For this review, take the finished solid that the model builds, in its own axes (mm). Face numbers are marked on the shaded views. A direction names the side the tool comes from. Coordinates: 2 decimals unless noted, no trailing zeros. Write each loop counter-clockwise with the first axis right and the second up, starting at its lowest first coordinate (ties: lowest second). Pieces come first, ordered by that corner, then holes. Notation, with made-up numbers: (6, 23.25) -> (33, 23.25) arc R20 ccw to (33, 57.25) -> close; hole circle Ø11 at (79, 35). An arc over 180 degrees is marked (long way). Put each result on its own line as item: value. Start each with the question number.
Item 1: Consider section B-B on x = 0. Give the boundary of the cut face in (y, z) (3 decimals), and give its area (3 significant figures).
Item 2: Consider section C-C on x = 23.5. Give the number of separate pieces and of enclosed holes in the cut face, and give its area (3 significant figures).
Item 3: Consider section A-A on y = 37.5. Give the boundary of the cut face in (x, z).
Item 4: Insertion check: P1, Ø8.5, axis at y = 24, z = 24, coming from the -X side; P2, Ø2.5, axis at x = -23.622, z = 23.622, coming from the +Y side; P3, Ø1, axis at x = -13.5, y = 37, coming from the +Z side; P4, Ø2.5, axis at x = -23, z = -24.5, coming from the +Y side. Each pin has a flat end and moves straight along its axis. Give the tip position at first contact, or say it passes through.
Item 5: To check wall thickness, follow L1, parallel to Z at x = 0, y = -0.9 (3 decimals); L2, parallel to Y at x = -16.5, z = 12.5; L3, parallel to X at y = 28.5, z = 24. State the ranges of each line that lie inside material, in increasing order.
Item 6: For the marked faces 1, 2 and 3, list the 3-axis set-ups (+Z, -Z, +X, -X, +Y, -Y) from which the entire face can be reached by the end or side of a thin tool; tool diameter is ignored.
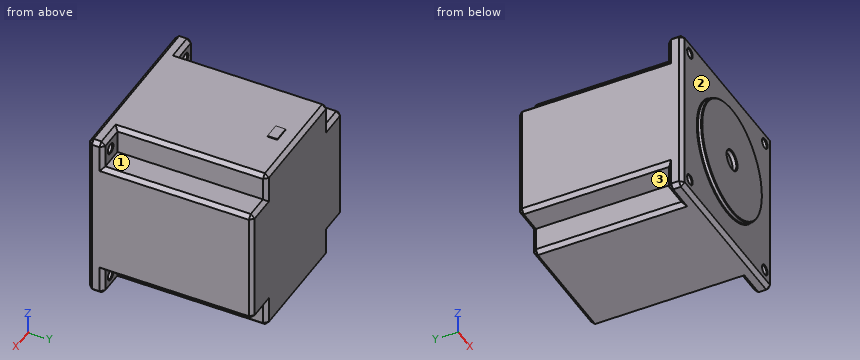
```python
from build123d import *

# Parameters (mm, degrees)
F0_W      = 56.388
F0_H      = 56.388
F0_R      = 1.4859
F0_R_2    = 19.05
F0_R_3    = 3.175
F1_DEPTH  = 54.102
F2_DEPTH  = 1.524
F3_DEPTH  = 20.32
F5_DEPTH  = 12.7
F6_W      = 8.89
F6_H      = 8.89
F7_DEPTH  = 49.022
F8_SIZE   = 1.27
F9_SIZE   = 0.254
F9_2_SIZE = 0.254
F10_W     = 5.2164322697
F10_H     = 3.265157342
F11_DEPTH = 0.254


with BuildPart() as f1:
    # F0 (on Front) → F1 (new body)
    with BuildSketch(Plane.XZ):
        Rectangle(F0_W, F0_H)
        with Locations((-23.622, -23.622)):
            Circle(F0_R, mode=Mode.SUBTRACT)
        with Locations((23.622, -23.622)):
            Circle(F0_R, mode=Mode.SUBTRACT)
        with Locations((-23.622, 23.622)):
            Circle(F0_R, mode=Mode.SUBTRACT)
        Circle(F0_R_2, mode=Mode.SUBTRACT)
        with Locations((23.622, 23.622)):
            Circle(F0_R, mode=Mode.SUBTRACT)
        Circle(F0_R_2)
        Circle(F0_R_3, mode=Mode.SUBTRACT)
        Circle(F0_R_3)
    extrude(amount=-F1_DEPTH)

    # F0 (on Front) → F2 (join)
    with BuildSketch(Plane.XZ):
        Circle(F0_R_2)
        Circle(F0_R_3, mode=Mode.SUBTRACT)
    extrude(amount=F2_DEPTH)

    # F6 (on face) → F7 (cut)
    with BuildSketch(Plane(origin=(0, 54.102, 0), x_dir=(-1, 0, 0), z_dir=(0, 1, 0))):
        with Locations((-23.749, 23.749)):
            Rectangle(F6_W, F6_H)
        with Locations((23.749, 23.749)):
            Rectangle(F6_W, F6_H)
        with Locations((23.749, -23.749)):
            Rectangle(F6_W, F6_H)
        with Locations((-23.749, -23.749)):
            Rectangle(F6_W, F6_H)
    extrude(amount=-F7_DEPTH, mode=Mode.SUBTRACT)

    # F8
    f8_edges = [f1.edges().sort_by_distance(p)[0] for p in [
        (-28.194, 0, 0),
        (-28.194, 2.54, -28.194),
        (-28.194, 5.08, -23.749),
        (-28.194, 29.591, -19.304),
        (-28.194, 54.102, 0),
        (-28.194, 29.591, 19.304),
        (-28.194, 5.08, 23.749),
        (-28.194, 2.54, 28.194),
        (0, 0, 28.194),
        (-23.749, 5.08, 28.194),
        (-19.304, 29.591, 28.194),
        (0, 54.102, 28.194),
        (19.304, 29.591, 28.194),
        (23.749, 5.08, 28.194),
        (28.194, 2.54, 28.194),
        (28.194, 0, 0),
        (28.194, 5.08, 23.749),
        (28.194, 29.591, 19.304),
        (28.194, 54.102, 0),
        (28.194, 29.591, -19.304),
        (28.194, 5.08, -23.749),
        (28.194, 2.54, -28.194),
        (0, 0, -28.194),
        (23.749, 5.08, -28.194),
        (19.304, 29.591, -28.194),
        (0, 54.102, -28.194),
        (-19.304, 29.591, -28.194),
        (-23.749, 5.08, -28.194),
        (23.749, 54.102, -19.304),
        (19.304, 54.102, -23.749),
        (-19.304, 54.102, -23.749),
        (-23.749, 54.102, -19.304),
        (-23.749, 54.102, 19.304),
        (-19.304, 54.102, 23.749),
        (19.304, 54.102, 23.749),
        (23.749, 54.102, 19.304),
    ]]
    chamfer(f8_edges, length=F8_SIZE)

    # F9
    f9_edges = [f1.edges().sort_by_distance(p)[0] for p in [
        (-25.1079, 5.08, 23.622),
        (-25.1079, 5.08, -23.622),
        (22.1361, 5.08, 23.622),
        (22.1361, 5.08, -23.622),
        (22.1361, 0, -23.622),
        (22.1361, 0, 23.622),
        (-25.1079, 0, 23.622),
        (-25.1079, 0, -23.622),
        (-19.05, 0, 0),
        (-19.05, -1.524, 0),
        (-3.175, -1.524, 0),
    ]]
    chamfer(f9_edges, length=F9_SIZE)

    # F10 (on face) → F11 (join)
    with BuildSketch(Plane.XY.offset(28.194)):
        with Locations((0, 47.2612604499)):
            Rectangle(F10_W, F10_H)
    extrude(amount=F11_DEPTH)


with BuildPart() as f3:
    # F0 (on Front) → F3 (new body)
    with BuildSketch(Plane.XZ):
        Circle(F0_R_3)
    extrude(amount=F3_DEPTH)

    # F4 (on face) → F5 (cut)
    with BuildSketch(Plane.XZ.offset(20.32)):
        with BuildLine():
            ThreePointArc((1.7989226109, 2.6162), (0, 3.175), (-1.7989226109, 2.6162))
            Line((-1.7989226109, 2.6162), (1.7989226109, 2.6162))
        make_face()
    extrude(amount=-F5_DEPTH, mode=Mode.SUBTRACT)

    # F9#2
    f9_2_edges = [f3.edges().sort_by_distance(p)[0] for p in [
        (-1.478013, -20.32, -2.81),
        (0, -20.32, 2.6162),
    ]]
    chamfer(f9_2_edges, length=F9_2_SIZE)


solid = f1.part
```
Return value:
1. outline: (-1.524, -18.796) -> (-1.27, -19.05) -> (-0.254, -19.05) -> (0, -19.304) -> (0, -26.924) -> (1.27, -28.194) -> (52.832, -28.194) -> (54.102, -26.924) -> (54.102, 26.924) -> (52.832, 28.194) -> (48.894, 28.194) -> (48.894, 28.448) -> (45.629, 28.448) -> (45.629, 28.194) -> (1.27, 28.194) -> (0, 26.924) -> (0, 19.304) -> (-0.254, 19.05) -> (-1.27, 19.05) -> (-1.524, 18.796) -> (-1.524, 3.429) -> (-1.27, 3.175) -> (0, 3.175) -> (0, -3.175) -> (-1.27, -3.175) -> (-1.524, -3.429) -> close
1. area: 3,100 mm^2
2. separate pieces: 3
2. enclosed holes: 0
2. area: 2,140 mm^2
3. outline: (-28.19, -18.03) -> (-26.92, -19.3) -> (-19.3, -19.3) -> (-19.3, -26.92) -> (-18.03, -28.19) -> (18.03, -28.19) -> (19.3, -26.92) -> (19.3, -19.3) -> (26.92, -19.3) -> (28.19, -18.03) -> (28.19, 18.03) -> (26.92, 19.3) -> (19.3, 19.3) -> (19.3, 26.92) -> (18.03, 28.19) -> (-18.03, 28.19) -> (-19.3, 26.92) -> (-19.3, 19.3) -> (-26.92, 19.3) -> (-28.19, 18.03) -> close
4. P1: x = -19.3
4. P2: through
4. P3: z = 28.19
4. P4: y = 5.08
5. L1: -19.05 to -3.175, 3.175 to 19.05
5. L2: 0 to 54.1
5. L3: -19.3 to 19.3
6. face 1: +Z, +X, +Y
6. face 2: -Y
6. face 3: -Z, -X, +Y
